Autodesk Inventor part; units mm, degrees
ref_plane "YZ Plane" through (0, 0, 0) normal (1, 0, 0) x (0, 1, 0)
ref_plane "XZ Plane" through (0, 0, 0) normal (0, 1, 0) x (-1, 0, 0)
ref_plane "XY Plane" through (0, 0, 0) normal (0, 0, 1) x (1, 0, 0)
sketch "Sketch1" plane through (0, 0, 0) normal (0, 0, 1) x (1, 0, 0)
  line L0 (-4.75, 2.9559) -> (0, 5.2945)
  line L1 (0, 5.2945) -> (4.75, 2.9559)
  line L2 (4.75, 2.9559) -> (4.75, -2.9559)
  line L3 (4.75, -2.9559) -> (0, -5.2945)
  line L4 (0, -5.2945) -> (-4.75, -2.9559)
  line L5 (-4.75, -2.9559) -> (-4.75, 2.9559)
  circle A0 centre (0, 0) radius 2.5
  circle A1 centre (0, 0) radius 4.75
  point P0 (4.75, 0)
  dimension "d6" = 5
  dimension "d8" = 9.5
extrude "Extrusion1" add sketch "Sketch1" along normal blind 4
properties part number "M5-nut"
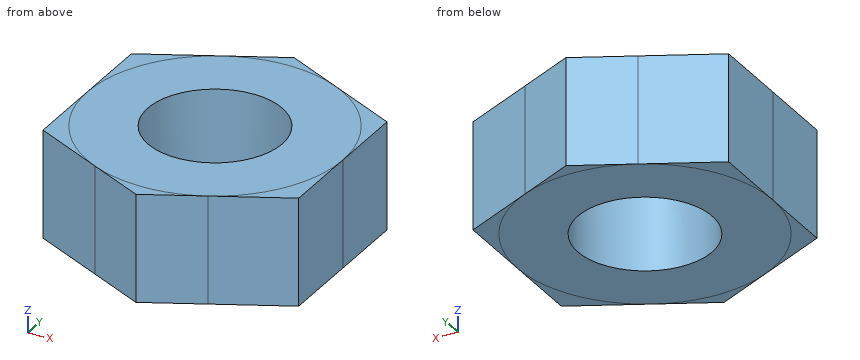
Can you work these out from the model? Positions are in its coordinate system, mm. Give positions to 0.01 mm unless a question says otherwise; leave off trailing zeros. Order: outer loops, then holes, each group sorted by start corner. A loop starts at its lowest first (then second) coordinate and runs counter-clockwise, first axis right, second up. Notation, with made-up numbers: (5, -36) - (56, -36) arc R26 ccw to (56, -7) - close; hole circle Ø6 at (45, 88). An arc over 180 degrees is marked (long way). Use a Markdown table: item, result. Add a question column.
Q1. If we section it at D-D on y = -4.5: Write out the boundary of the cut face in (x, z).
Q2. If we section it at A-A on y = -1.5: Write out the boundary of the cut face in (x, z), plus the area to 3 significant figures.
Q3. If we section it at B-B on z = 1.3: Write out the boundary of the cut face in (x, y).
Q4. Please list where these lines run through material, in increasing order: line 1 along Y through (x, z) = (2.25, 0.45); line 2 along X through (y, z) = (-2.25, 0.2); line 3 along X through (y, z) = (2, 3.7).
Q5. If we section it at C-C on x = 1.25: Write out the boundary of the cut face in (y, z), plus the area to 3 significant figures.
Answers follow:
| question | item | result |
|---|---|---|
| 1 | outline | (-1.61, 0) - (1.61, 0) - (1.61, 4) - (-1.61, 4) - close |
| 2 | outline | (-4.75, 0) - (-2, 0) - (-2, 4) - (-4.75, 4) - close; (2, 0) - (4.75, 0) - (4.75, 4) - (2, 4) - close |
| 2 | area | 22.0 mm^2 |
| 3 | outline | (-4.75, -2.96) - (0, -5.29) - (4.75, -2.96) - (4.75, 2.96) - (0, 5.29) - (-4.75, 2.96) - close; hole circle Ø5 at (0, 0) |
| 4 | line 1 | y = -4.19 to -1.09, 1.09 to 4.19 |
| 4 | line 2 | x = -4.75 to -1.09, 1.09 to 4.75 |
| 4 | line 3 | x = -4.75 to -1.5, 1.5 to 4.75 |
| 5 | outline | (-4.68, 0) - (-2.17, 0) - (-2.17, 4) - (-4.68, 4) - close; (2.17, 0) - (4.68, 0) - (4.68, 4) - (2.17, 4) - close |
| 5 | area | 20.1 mm^2 |
